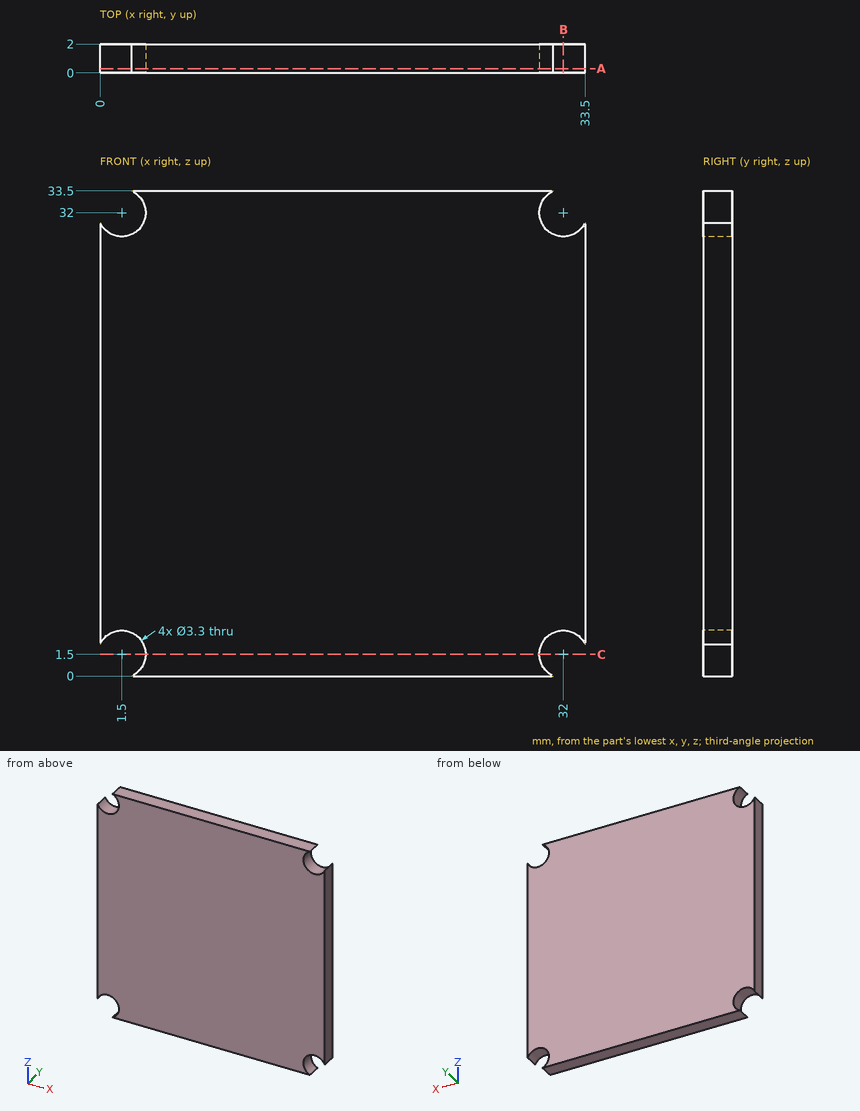
Job drawing, mm, ordinate dimensions from the low corner. One solid piece. Give positions to 0.01 mm unless a question says otherwise; leave off trailing zeros. Write each loop counter-clockwise with the first axis right and the second up, starting at its lowest first coordinate (ties: lowest second). Pieces come first, ordered by that corner, then holes. Notation, with made-up numbers: M 71,5 L 82,5 A23 cw 82,39 Z; hole C 55,82 d11. An arc over 180 degrees is marked long. One line per item, written item: value. Start each with the question number.
Q1. Saw through at A-A, the plane y = 0.3. Write the cut outline in (x, z), plus the area to 3 significant figures.
Q2. Drop flat-ended pins along their axis: pin 1 Ø4 at (x, z) = (32, 32) entering from +Y; pin 2 Ø2 at (x, z) = (1.5, 1.5) entering from +Y. Give the stop position or say it passes through.
Q3. Probe probe 1 along X at (y, z) = (1, 1.5). List the from-to ranges inside material, lowest first. Write a range as [from, to].
Q4. Saw through at B-B, the plane x = 32. Write the cut outline in (y, z), plus the area to 3 significant figures.
Q5. Saw through at C-C, the plane z = 1.5. Write the cut outline in (x, y), plus the area to 3 significant figures.
Output values:
1. outline: M 0,2.19 A1.65 cw long 2.19,0 L 31.31,0 A1.65 cw long 33.5,2.19 L 33.5,31.31 A1.65 cw long 31.31,33.5 L 2.19,33.5 A1.65 cw long 0,31.31 Z
1. area: 1,090 mm²
2. pin 1: stops at y = 2
2. pin 2: passes through
3. probe 1: x = [3.15, 30.35]
4. outline: M 0,3.15 L 2,3.15 L 2,30.35 L 0,30.35 Z
4. area: 54.4 mm²
5. outline: M 3.15,0 L 30.35,0 L 30.35,2 L 3.15,2 Z
5. area: 54.4 mm²
